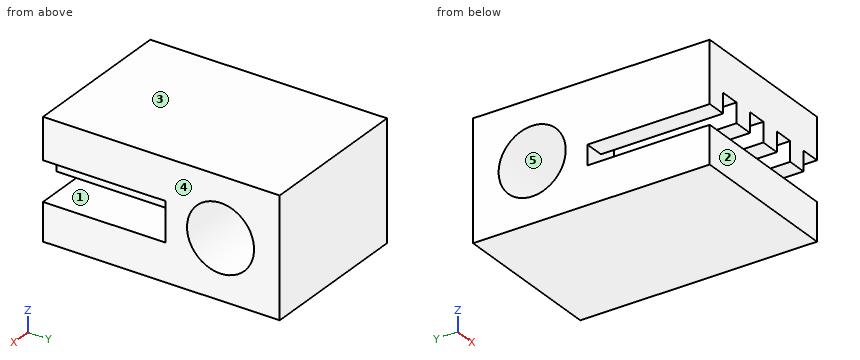
from build123d import *

# Parameters (mm, degrees)
F0_W     = 8
F0_H     = 12
F1_DEPTH = 6
F3_DEPTH = 6.2
F4_R     = 1.7
F5_DEPTH = 25


with BuildPart() as f1:
    # F0 (on Top) → F1 (new body)
    with BuildSketch(Plane.XY):
        with Locations((10.135715, 1.112354)):
            Rectangle(F0_W, F0_H)
    extrude(amount=F1_DEPTH)

    # F2 (on face) → F3 (cut)
    with BuildSketch(Plane.XZ.offset(4.887646)):
        Polygon((6.135715, 2.910965), (6.135715, 1.910965), (14.135715, 1.910965), (14.135715, 2.910965), (14.135715, 3.910965), (13.135715, 3.910965), (13.135715, 2.910965), (12.135715, 2.910965), (12.135715, 3.910965), (11.135715, 3.910965), (11.135715, 2.910965), (10.135715, 2.910965), (10.135715, 3.910965), (9.135715, 3.910965), (9.135715, 2.910965), (8.135715, 2.910965), (8.135715, 3.910965), (7.135715, 3.910965), (7.135715, 2.910965), align=None)
    extrude(amount=-F3_DEPTH, mode=Mode.SUBTRACT)

    # F4 (on face) → F5 (cut)
    with BuildSketch(Plane(origin=(6.135715, 0, 0), x_dir=(0, -1, 0), z_dir=(-1, 0, 0))):
        with Locations((-4.112354, 3)):
            Circle(F4_R)
    extrude(amount=-F5_DEPTH, mode=Mode.SUBTRACT)


solid = f1.part
CAD build for the part. Positions are in the model's coordinates, mm. Face numbers are marked on the shaded views. A direction names the side the tool comes from. Round coordinates to 2 decimals unless told otherwise and drop trailing zeros. Write each loop counter-clockwise with the first axis right and the second up, starting at its lowest first coordinate (ties: lowest second). Pieces come first, ordered by that corner, then holes. Notation, with made-up numbers: M 9,63.25 L 67,63.25 A29 cw 67,94.25 Z; hole C -8,-1.75 d8. An arc over 180 degrees is marked long. Put each result on its own line as item: value. Start each with the question number.
1) Saw through at C-C, the plane z = 1.6. Write the cut outline in (x, y).
2) Saw through at A-A, the plane y = -0.5. Write the cut outline in (x, z), and give its area (3 significant figures).
3) Saw through at D-D, the plane y = 5. Write the cut outline in (x, z).
4) 3-axis set-ups, long thin cutter, end or side, ignore diameter. For the marked faces 1 and 2: which of +Z, -Z, +X, -X, +Y, -Y reach the whole face in a straight line?
5) Pull direction Z, two halves, no side cores. Call the marked faces 3, 4 and 5: pulls with the +Z half, pulls with the -Z half, needs draft (parallel to the pull), parting line crosses it, or undercut.
6) Drill centre lines: probe 1 along Z at (x, y) = (8.5, -3); probe 2 along X at (y, z) = (0.75, 3.5); probe 3 along Z at (x, y) = (13.5, 0.25). Where is each one in solid material? Low to high. Write a range as [from, to].
7) Saw through at B-B, the plane x = 12. Write the cut outline in (y, z), and give its area (3 significant figures).
Resolved:
1. outline: M 6.14,-4.89 L 14.14,-4.89 L 14.14,3.15 L 6.14,3.15 Z; M 6.14,5.08 L 14.14,5.08 L 14.14,7.11 L 6.14,7.11 Z
2. outline: M 6.14,0 L 14.14,0 L 14.14,1.91 L 6.14,1.91 Z; M 6.14,2.91 L 7.14,2.91 L 7.14,3.91 L 8.14,3.91 L 8.14,2.91 L 9.14,2.91 L 9.14,3.91 L 10.14,3.91 L 10.14,2.91 L 11.14,2.91 L 11.14,3.91 L 12.14,3.91 L 12.14,2.91 L 13.14,2.91 L 13.14,3.91 L 14.14,3.91 L 14.14,6 L 6.14,6 Z
2. area: 36.0 mm²
3. outline: M 6.14,0 L 14.14,0 L 14.14,1.55 L 6.14,1.55 Z; M 6.14,4.45 L 14.14,4.45 L 14.14,6 L 6.14,6 Z
4. face 1: +X, -X, -Y
4. face 2: +Z, -Z, +X, -X, -Y
5. face 3: pulls with the +Z half
5. face 4: needs draft
5. face 5: undercut
6. probe 1: [0, 1.91], [2.91, 6]
6. probe 2: [6.14, 7.14], [8.14, 9.14], [10.14, 11.14], [12.14, 13.14]
6. probe 3: [0, 1.91], [3.91, 6]
7. outline: M -4.89,0 L 7.11,0 L 7.11,6 L -4.89,6 L -4.89,3.91 L 1.31,3.91 L 1.31,1.91 L -4.89,1.91 Z; hole C 4.11,3 d3.4
7. area: 50.5 mm²
